Could you check a few things on this model? Use its own coordinates, in mm. A direction names the side the tool comes from. Round coordinates to 2 decimals unless told otherwise and drop trailing zeros. Loops run counter-clockwise (first coordinate to the right, second up) from the corner with the lowest first, then second, coordinate; pieces in that order, holes last. Notation, with made-up numbers: (80.5, -21.5) - (132.5, -21.5) arc R27 cw to (132.5, 16.5) - close; hole circle Ø8 at (63.25, 37). An arc over 180 degrees is marked (long way). Answer as CSV lines item,"result". Start each with the question number.
1) Suppose I cut it at A-A, the plane z = 11. Write out the boundary of the cut face in (x, y).
2) Suppose I cut it at D-D, the plane y = 0. Write out the boundary of the cut face in (x, z).
3) Suppose I cut it at C-C, the plane x = 4. Write out the boundary of the cut face in (y, z).
4) Which directions (+Z, -Z, +X, -X, +Y, -Y) give clear straight access to the entire face, cutting with the end or side of a thin tool? Please do faces 5 (the face through (-15, -20, 7)), 6 (the face through (0, -13, 9)), 7 (the face through (0, -13.5, 1)).
5) We'd pull the mould along X, two halves only. Please class faces 1 (the face through (-2, -14, 0)), 2 (the face through (0, -15, 11)), 3 (the face through (-26.5, 0, 7)), 4 (the face through (23.5, 0, 7)): pulls with the +X half, pulls with the -X half, needs draft (parallel to the pull), parting line crosses it, or undercut.
6) I'm going to push flat-ended pins straight in: pin 1 Ø7.5 at (y, z) = (-20, 6) entering from +X; pin 2 Ø5 at (y, z) = (-22, 8.5) entering from -X; pin 3 Ø6 at (x, y) = (-4.5, 8.5) entering from -Z. Where does each tip first touch, or does it pass through?
7) Please list where these lines run through material, in increasing order: line 1 along Y through (x, z) = (-2, 10); line 2 along Y through (x, z) = (18.5, 5); line 3 along Y through (x, z) = (-13, 12.6).
8) Suppose I cut it at B-B, the plane x = 13. Write out the boundary of the cut face in (y, z).
```python
from build123d import *

# Parameters (mm, degrees)
SKETCH1_W           = 53
SKETCH1_H           = 30
BOSS_EXTRUDE1_DEPTH = 15
SKETCH2_R           = 8.25
CUT_EXTRUDE1_DEPTH  = 16
SKETCH3_W           = 47
SKETCH3_H           = 24
CUT_EXTRUDE2_DEPTH  = 12
SKETCH4_W           = 15
SKETCH4_H           = 6
CUT_EXTRUDE3_DEPTH  = 12
SKETCH6_W           = 50
SKETCH6_H           = 27
CUT_EXTRUDE4_DEPTH  = 1.5
SKETCH7_W           = 30
SKETCH7_H           = 10
BOSS_EXTRUDE2_DEPTH = 10
SKETCH8_W           = 24
SKETCH8_H           = 7
CUT_EXTRUDE5_DEPTH  = 13.5
SKETCH9_R           = 2.25
CUT_EXTRUDE6_DEPTH  = 4


with BuildPart() as part:
    # Sketch1 → Boss-Extrude1 (new body)
    with BuildSketch(Plane.XY):
        Rectangle(SKETCH1_W, SKETCH1_H)
    extrude(amount=BOSS_EXTRUDE1_DEPTH)

    # Sketch2 → Cut-Extrude1 (cut, through all)
    with BuildSketch(Plane.XY.offset(15)):
        with Locations((13, 0)):
            Circle(SKETCH2_R)
        with Locations((-13, 0)):
            Circle(SKETCH2_R)
    extrude(amount=-CUT_EXTRUDE1_DEPTH, mode=Mode.SUBTRACT)

    # Sketch3 → Cut-Extrude2 (cut)
    with BuildSketch(Plane(origin=(0, 0, 0), x_dir=(-1, 0, 0), z_dir=(0, 0, -1))):
        Rectangle(SKETCH3_W, SKETCH3_H)
    extrude(amount=-CUT_EXTRUDE2_DEPTH, mode=Mode.SUBTRACT)

    # Sketch4 → Cut-Extrude3 (cut)
    with BuildSketch(Plane(origin=(0, -12, 0), x_dir=(1, 0, 0), z_dir=(0, 1, 0))):
        with Locations((0, -6)):
            Rectangle(SKETCH4_W, SKETCH4_H)
    extrude(amount=-CUT_EXTRUDE3_DEPTH, mode=Mode.SUBTRACT)

    # Sketch6 → Cut-Extrude4 (cut)
    with BuildSketch(Plane(origin=(0, 0, 0), x_dir=(-1, 0, 0), z_dir=(0, 0, -1))):
        Rectangle(SKETCH6_W, SKETCH6_H)
    extrude(amount=-CUT_EXTRUDE4_DEPTH, mode=Mode.SUBTRACT)

    # Sketch7 → Boss-Extrude2 (add)
    with BuildSketch(Plane.XZ.offset(15)):
        with Locations((0, 7.5)):
            Rectangle(SKETCH7_W, SKETCH7_H)
    extrude(amount=BOSS_EXTRUDE2_DEPTH)

    # Sketch8 → Cut-Extrude5 (cut, through all)
    with BuildSketch(Plane.XY.offset(12.5)):
        with Locations((0, -18.5)):
            Rectangle(SKETCH8_W, SKETCH8_H)
    extrude(amount=-CUT_EXTRUDE5_DEPTH, mode=Mode.SUBTRACT)

    # Sketch9 → Cut-Extrude6 (cut)
    with BuildSketch(Plane.XZ.offset(25)):
        with Locations((0, 7.5)):
            Circle(SKETCH9_R)
    extrude(amount=-CUT_EXTRUDE6_DEPTH, mode=Mode.SUBTRACT)


solid = part.part
```
Filled sheet:
1,outline,"(-26.5, -15) - (-15, -15) - (-15, -25) - (15, -25) - (15, -15) - (26.5, -15) - (26.5, 15) - (-26.5, 15) - close; hole (-23.5, -12) - (23.5, -12) - (23.5, 12) - (-23.5, 12) - close; hole (-12, -22) - (12, -22) - (12, -15) - (-12, -15) - close"
2,outline,"(-26.5, 0) - (-25, 0) - (-25, 1.5) - (-23.5, 1.5) - (-23.5, 12) - (-21.25, 12) - (-21.25, 15) - (-26.5, 15) - close; (-4.75, 12) - (4.75, 12) - (4.75, 15) - (-4.75, 15) - close; (21.25, 12) - (23.5, 12) - (23.5, 1.5) - (25, 1.5) - (25, 0) - (26.5, 0) - (26.5, 15) - (21.25, 15) - close"
3,outline,"(-25, 2.5) - (-22, 2.5) - (-22, 12.5) - (-25, 12.5) - close; (-15, 0) - (-13.5, 0) - (-13.5, 1.5) - (-12, 1.5) - (-12, 3) - (-15, 3) - close; (-15, 9) - (-12, 9) - (-12, 12) - (12, 12) - (12, 1.5) - (13.5, 1.5) - (13.5, 0) - (15, 0) - (15, 15) - (-15, 15) - close"
4,face 5,"+Z, -Z, -X, -Y"
4,face 6,"none"
4,face 7,"-Z"
5,face 1,"needs draft"
5,face 2,"undercut"
5,face 3,"pulls with the -X half"
5,face 4,"undercut"
6,pin 1,"x = 15"
6,pin 2,"x = -15"
6,pin 3,"z = 12"
7,line 1,"-25 to -22, -15 to -12, 12 to 15"
7,line 2,"-15 to -12, 12 to 15"
7,line 3,"-15 to -8.25, 8.25 to 15"
8,outline,"(-25, 2.5) - (-15, 2.5) - (-15, 0) - (-13.5, 0) - (-13.5, 1.5) - (-12, 1.5) - (-12, 12) - (-8.25, 12) - (-8.25, 15) - (-15, 15) - (-15, 12.5) - (-25, 12.5) - close; (8.25, 12) - (12, 12) - (12, 1.5) - (13.5, 1.5) - (13.5, 0) - (15, 0) - (15, 15) - (8.25, 15) - close"
